from build123d import *

# Parameters (mm, degrees)
F0_R     = 10
F1_DEPTH = 25
F2_DEPTH = 50
F3_SIZE  = 2


with BuildPart() as f1:
    # F0 (on Front) → F1 (new body)
    with BuildSketch(Plane.XZ):
        with BuildLine():
            ThreePointArc((2.777778, -24.8452), (18.6339, -16.666667), (25, 0))
            ThreePointArc((25, 0), (18.6339, 16.666667), (2.777778, 24.8452))
            ThreePointArc((2.777778, 24.8452), (-25, 0), (2.777778, -24.8452))
        make_face()
        Circle(F0_R, mode=Mode.SUBTRACT)
        with BuildLine():
            ThreePointArc((2.777778, 24.8452), (18.6339, 16.666667), (25, 0))
            ThreePointArc((25, 0), (18.6339, -16.666667), (2.777778, -24.8452))
            Line((2.777778, -24.8452), (91.666667, -14.90712))
            ThreePointArc((91.666667, -14.90712), (75, 0), (91.666667, 14.90712))
            Line((91.666667, 14.90712), (2.777778, 24.8452))
        make_face()
        with BuildLine():
            ThreePointArc((105, 0), (101.18034, 10), (91.666667, 14.90712))
            ThreePointArc((91.666667, 14.90712), (75, 0), (91.666667, -14.90712))
            ThreePointArc((91.666667, -14.90712), (101.18034, -10), (105, 0))
        make_face()
        with Locations((90, 0)):
            Circle(F0_R, mode=Mode.SUBTRACT)
    extrude(amount=F1_DEPTH)

    # F0 (on Front) → F2 (join)
    with BuildSketch(Plane.XZ):
        with BuildLine():
            ThreePointArc((2.777778, -24.8452), (18.6339, -16.666667), (25, 0))
            ThreePointArc((25, 0), (18.6339, 16.666667), (2.777778, 24.8452))
            ThreePointArc((2.777778, 24.8452), (-25, 0), (2.777778, -24.8452))
        make_face()
        Circle(F0_R, mode=Mode.SUBTRACT)
    extrude(amount=F2_DEPTH)

    # F3
    f3_edges = [f1.edges().sort_by_distance(p)[0] for p in [
        (-10, -50, 0),
        (-10, 0, 0),
        (-2.777778, -50, 24.8452),
        (80, 0, 0),
        (80, -25, 0),
    ]]
    chamfer(f3_edges, length=F3_SIZE)


solid = f1.part
Geometry check sheet. Reference: the model listing, model coordinates, mm. Coordinates: 2 decimals unless noted, no trailing zeros. Order: outer loops, then holes, each group sorted by start corner. A loop starts at its lowest first (then second) coordinate and runs counter-clockwise, first axis right, second up. Notation, with made-up numbers: (47.5, 80.5) - (72.5, 80.5) arc R13 cw to (72.5, 105.5) - close; hole circle Ø2 at (26, -17). An arc over 180 degrees is marked (long way). Answer in a Markdown table with one row per item. Add a question column.
1) Release check for a two-part mould opening along X. For faces 1 (the flat face through (47.844, -12.325, 19.807)), 2 (the flat face through (39, 0, 0)), 3 (the conical face through (-2.195, -48.125, -9.884)), 4 (the conical face through (81.965, -23.125, -6.161)) record: +X half, -X half, draft (parallel to the pull), parting line (faces both ways), or undercut.
2) Gauge pin test, flat ends, axial feed: P1, Ø1, axis at y = -32, z = -1, coming from the +X side (3 decimals); P2, Ø12, axis at x = 80, y = -21.5, coming from the +Z side; P3, Ø2, axis at y = -13.5, z = 14.5, coming from the -X side; P4, Ø16, axis at x = 90, z = 0, coming from the +Y side. Record the tip position at first contact, or that the pin passes through.
3) Cross-section at A-A, the plane x = 0. Record the cut outline in (y, z).
4) Material ranges on line 1 along Z through (x, y) = (0, -33); line 2 along Y through (x, z) = (74, -3); line 3 along Z through (x, y) = (85.5, -20.5), recorded low to high. Write a range as [from, to].
5) Cross-section at B-B, the plane y = -12. Record the cut outline in (x, z).
6) Cross-section at C-C, the plane y = -34. Record the cut outline in (x, z), then the cut area to 3 significant figures.
7) Cross-section at D-D, the plane z = 3. State how many separate pieces and enclosed holes the cut face has, then the cut area to 3 significant figures.
Check result:
| question | item | result |
|---|---|---|
| 1 | face 1 | +X half |
| 1 | face 2 | draft |
| 1 | face 3 | undercut |
| 1 | face 4 | undercut |
| 2 | P1 | stops at x = 24.995 |
| 2 | P2 | stops at z = 16.88 |
| 2 | P3 | stops at x = -21.04 |
| 2 | P4 | passes through |
| 3 | outline | (-50, -23) - (-48, -25) - (0, -25) - (0, -12) - (-2, -10) - (-48, -10) - (-50, -12) - close; (-50, 12) - (-48, 10) - (-2, 10) - (0, 12) - (0, 25) - (-48, 25) - (-50, 23) - close |
| 4 | line 1 | z = [-25, -10], [10, 25] |
| 4 | line 2 | y = [-25, 0] |
| 4 | line 3 | z = [-15.6, -8.93], [8.93, 15.6] |
| 5 | outline | (2.78, -24.85) - (91.67, -14.91) arc R15 ccw to (91.67, 14.91) - (2.78, 24.85) arc R25 ccw (long way) to start; hole circle Ø20 at (0, 0); hole circle Ø20 at (90, 0) |
| 6 | outline | (2.78, 24.85) arc R25 ccw (long way) to (25, 0) arc R25 ccw to start; hole circle Ø20 at (0, 0) |
| 6 | area | 1,650 mm² |
| 7 | separate pieces | 3 |
| 7 | enclosed holes | 0 |
| 7 | area | 3,030 mm² |
